Geometry check sheet. Reference: the model listing, model coordinates, mm. A direction names the side the tool comes from. Give positions to 0.01 mm unless a question says otherwise; leave off trailing zeros. Order: outer loops, then holes, each group sorted by start corner. A loop starts at its lowest first (then second) coordinate and runs counter-clockwise, first axis right, second up.
from build123d import *

# Parameters (mm, degrees)
SKETCH_1_W          = 215
SKETCH_1_H          = 114
EXTRUDE_1_DEPTH     = 50
SKETCH_2_W          = 22.304316617
SKETCH_2_H          = 103.168471384
CUT_EXTRUDE_1_DEPTH = 40
SKETCH_3_R          = 2
CUT_EXTRUDE_2_DEPTH = 4


with BuildPart() as part:
    # 草图1 → 凸台-拉伸1 (new body)
    with BuildSketch(Plane(origin=(0, 0, 0), x_dir=(0, 0, -1), z_dir=(1, 0, 0))):
        with Locations((-107.5, 57)):
            Rectangle(SKETCH_1_W, SKETCH_1_H)
    extrude(amount=EXTRUDE_1_DEPTH)

    # 草图2 → 切除-拉伸1 (cut)
    with BuildSketch(Plane.ZY):
        with Locations((11.152158309, 57.116706416)):
            Rectangle(SKETCH_2_W, SKETCH_2_H)
    extrude(amount=-CUT_EXTRUDE_1_DEPTH, mode=Mode.SUBTRACT)

    # 草图3 → 切除-拉伸2 (cut)
    with BuildSketch(Plane(origin=(50, 0, 0), x_dir=(0, 0, -1), z_dir=(1, 0, 0))):
        with Locations((-182.5, 82)):
            Circle(SKETCH_3_R)
        with Locations((-32.5, 82)):
            Circle(SKETCH_3_R)
        with Locations((-32.5, 32)):
            Circle(SKETCH_3_R)
        with Locations((-182.5, 32)):
            Circle(SKETCH_3_R)
    extrude(amount=-CUT_EXTRUDE_2_DEPTH, mode=Mode.SUBTRACT)


solid = part.part
Item 1: Set-up check for faces 1 (the flat face through (25, 56, 215)), 2 (the flat face through (20, 56, 22.304)), 3 (the flat face through (46, 32, 33)): record each of +Z, -Z, +X, -X, +Y, -Y from which the full face is reachable in a straight line by a thin tool's end or side.
Reported:
face 1: +Z, +X, -X, +Y, -Y
face 2: -Z, -X
face 3: +X
Item 2: Scan lines: L1, parallel to Y at x = 47.8, z = 182.5; L2, parallel to Y at x = 47, z = 182; L3, parallel to Z at x = 26, y = 60.5. Record each from-to range of solid material in increasing order.
Reported:
L1: y = 0 to 30, 34 to 80, 84 to 114
L2: y = 0 to 30.06, 33.94 to 80.06, 83.94 to 114
L3: z = 22.3 to 215
Item 3: Sectioned sample at C-C (y = 32). Enter the section's corners in (x, z), and give its area (3 significant figures).
Reported:
outline: (0, 22.3) - (40, 22.3) - (40, 0) - (50, 0) - (50, 30.5) - (46, 30.5) - (46, 34.5) - (50, 34.5) - (50, 180.5) - (46, 180.5) - (46, 184.5) - (50, 184.5) - (50, 215) - (0, 215) - close
area: 9,830 mm2
Item 4: Draft check along Y on faces 4 (the flat face through (0, 58, 109)), 5 (the flat face through (46, 82, 33)), 6 (the flat face through (40, 58, 11)), 7 (the flat face through (25, 0, 109)). Enter one of: released by +Y, released by -Y, zero draft, split by the parting line, or undercut.
Reported:
face 4: zero draft
face 5: undercut
face 6: undercut
face 7: released by -Y
Item 5: Sectioned sample at B-B (x = 24). Enter the section's corners in (y, z).
Reported:
outline: (0, 0) - (5.53, 0) - (5.53, 22.3) - (108.7, 22.3) - (108.7, 0) - (114, 0) - (114, 215) - (0, 215) - close
Item 6: Sectioned sample at A-A (y = 45). Enter the section's corners in (x, z), and give its area (3 significant figures).
Reported:
outline: (0, 22.3) - (40, 22.3) - (40, 0) - (50, 0) - (50, 215) - (0, 215) - close
area: 9,860 mm2
Item 7: Gauge pin test, flat ends, axial feed: pin 1 (1 mm diameter, centred on x = 33, y = 45, fed in from -Z); pin 2 (6.5 mm diameter, centred on y = 69, z = 7.5, fed in from -X); pin 3 (1.2 mm diameter, centred on y = 82, z = 183, fed in from +X). Record the tip position at first contact, or that the pin passes through.
Reported:
pin 1: stops at z = 22.3
pin 2: stops at x = 40
pin 3: stops at x = 46
